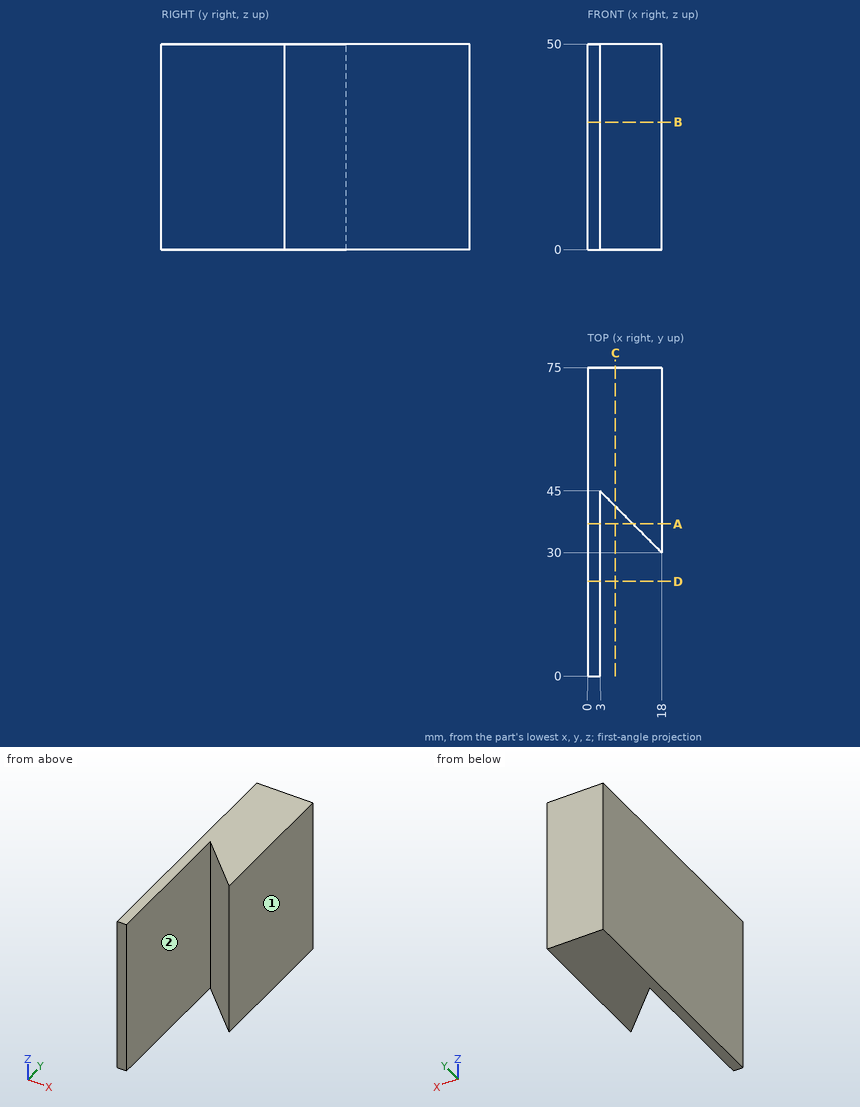
The figure shows three views and two pictorial views of one solid part (mm, origin at its lowest corner). Answer the questions. A direction names the side the tool comes from. Coordinates: 2 decimals unless noted, no trailing zeros. Loops run counter-clockwise (first coordinate to the right, second up) from the corner with the lowest first, then second, coordinate; pieces in that order, holes last. Notation, with made-up numbers: (-7.75, 15.5) -> (50.25, 15.5) arc R15 cw to (50.25, 19.5) -> close; hole circle Ø10 at (80, 16). An arc over 180 degrees is marked (long way). Use one line per item in the form item = value. Start each with the question number.
Item 1: Flat-ended cylindrical pins translate along their axes: pin 1 Ø2 at (y, z) = (48.5, 36) entering from -X; pin 2 Ø1.5 at (x, z) = (6.5, 44.5) entering from -Y. Find the tip coordinate at first contact, or state that the pin passes through.
Item 2: The part is cut by section D-D on y = 23. Determine the outline of the cut face in (x, z).
Item 3: The part is cut by section C-C on x = 6.75. Determine the outline of the cut face in (y, z).
Item 4: The part is cut by section A-A on y = 37. Determine the outline of the cut face in (x, z), then the cut area to 3 significant figures.
Item 5: Consider L1, parallel to X at y = 21.5, z = 26.5; L2, parallel to Y at x = 9.25, z = 45.5; L3, parallel to Y at x = 8, z = 29.5. Determine where each line is inside the solid, lowest interval first. Write a range as [from, to].
Item 6: A tool of negligible diameter and unlimited length cuts with its end or side. For the marked faces 1 and 2, from which of +Z, -Z, +X, -X, +Y, -Y can it reach the whole face along a straight path? Write none if from no direction.
Item 7: The part is cut by section B-B on z = 31. Determine the outline of the cut face in (x, y).
Answer key:
q1.pin_1 = 0
q1.pin_2 = 40.75
q2.outline = (0, 0) -> (3, 0) -> (3, 50) -> (0, 50) -> close
q3.outline = (41.25, 0) -> (75, 0) -> (75, 50) -> (41.25, 50) -> close
q4.outline = (0, 0) -> (3, 0) -> (3, 50) -> (0, 50) -> close; (11, 0) -> (18, 0) -> (18, 50) -> (11, 50) -> close
q4.area = 500 mm2
q5.L1 = [0, 3]
q5.L2 = [38.75, 75]
q5.L3 = [40, 75]
q6.face_1 = +Z, -Z, +X, +Y, -Y
q6.face_2 = +Z, -Z, -Y
q7.outline = (0, 0) -> (3, 0) -> (3, 45) -> (18, 30) -> (18, 75) -> (0, 75) -> close
